Can you work these out from the model? Positions are in its coordinate system, mm. Face numbers are marked on the shaded views. A direction names the side the tool comes from. Give positions to 0.01 mm unless a question says otherwise; leave off trailing zeros. Order: outer loops, then holes, each group sorted by start corner. A loop starts at its lowest first (then second) coordinate and runs counter-clockwise, first axis right, second up. Notation, with made-up numbers: (22, 58.5) - (74, 58.5) arc R24 ccw to (74, 92.5) - close; hole circle Ø9 at (-11.5, 79.25). An arc over 180 degrees is marked (long way). One line per question, with ' | ' between items.
```python
from build123d import *


with BuildPart() as part:
    # Sketch1 → Revolve1 (revolve)
    with BuildSketch(Plane.XY):
        with BuildLine():
            Line((0, 4.6), (0, 3.375))
            Line((0, 3.375), (1.35, 3.375))
            Line((1.35, 3.375), (1.35, 4.5))
            Line((1.35, 4.5), (4.65, 4.5))
            Line((4.65, 4.5), (4.65, 3.375))
            Line((4.65, 3.375), (6, 3.375))
            Line((6, 3.375), (6, 4.6))
            ThreePointArc((6, 4.6), (5.882842712, 4.882842712), (5.6, 5))
            Line((5.6, 5), (0.4, 5))
            ThreePointArc((0.4, 5), (0.117157288, 4.882842712), (0, 4.6))
        make_face()
    revolve(axis=Axis((50, 0, 0), (-1, 0, 0)))


solid = part.part
```
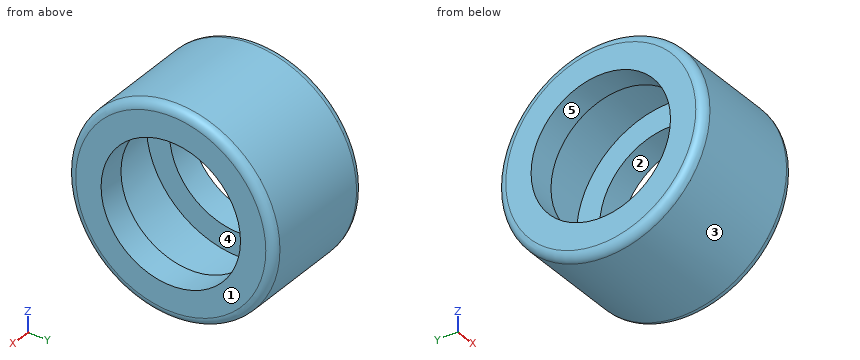
(1) Imagine slicing it at B-B (x = 1.15). List the corners of the cut face in (y, z) for me (3 decimals).
Answer below:
outline: circle Ø10 at (0, 0); hole circle Ø6.75 at (0, 0)
(2) Imagine slicing it at A-A (y = 0). List the corners of the cut face in (x, z) for me (3 decimals).
Answer below:
outline: (0, -4.6) arc R0.4 ccw to (0.4, -5) - (5.6, -5) arc R0.4 ccw to (6, -4.6) - (6, -3.375) - (4.65, -3.375) - (4.65, -4.5) - (1.35, -4.5) - (1.35, -3.375) - (0, -3.375) - close; (0, 3.375) - (1.35, 3.375) - (1.35, 4.5) - (4.65, 4.5) - (4.65, 3.375) - (6, 3.375) - (6, 4.6) arc R0.4 ccw to (5.6, 5) - (0.4, 5) arc R0.4 ccw to (0, 4.6) - close
(3) If I drill on line 1 (Z direction, x = 2.4, y = 0); line 2 (X direction, y = 0, z = 3.5); line 3 (Z direction, x = 5.65, y = 0) (3 decimals), over which ranges is the centre line in solid material (lowest first)?
Answer below:
line 1: -5 to -4.5, 4.5 to 5 | line 2: 0 to 1.35, 4.65 to 6 | line 3: -4.997 to -3.375, 3.375 to 4.997
(4) If we mould it in two halves opening along Y, with no side actions, what happens to the marked faces 1, 2 and 3? For each: released by +Y, released by -Y, zero draft, split by the parting line, or undercut.
Answer below:
face 1: zero draft | face 2: undercut | face 3: split by the parting line
(5) Will these pins go through, and if not, where does the flat tip stop? pin 1 (6 mm diameter, centred on y = -2.5, z = -2, fed in from +X); pin 2 (2 mm diameter, centred on x = 1.5, z = -1.5, fed in from -Y); pin 3 (4 mm diameter, centred on y = 0, z = 0, fed in from +X).
Answer below:
pin 1: x = 6 | pin 2: y = -4.97 | pin 3: through
(6) On a 3-axis mill with a long thin cutter (end or side, diameter ignored), from which of +Z, -Z, +X, -X, +Y, -Y can I reach the whole of each face in a straight line? I mean the marked faces 4 and 5. Say none if no direction works.
Answer below:
face 4: none | face 5: +X, -X
(7) Imagine slicing it at C-C (x = 4.35). List the corners of the cut face in (y, z) for me, and give its area (3 significant figures).
Answer below:
outline: circle Ø10 at (0, 0); hole circle Ø9 at (0, 0) | area: 14.9 mm^2
